Can you work these out from the model? Positions are in its coordinate system, mm. Face numbers are marked on the shaded views. A direction names the side the tool comes from. Round coordinates to 2 decimals unless told otherwise and drop trailing zeros. Write each loop counter-clockwise with the first axis right and the second up, starting at its lowest first coordinate (ties: lowest second). Pieces come first, ordered by that corner, then holes. Notation, with made-up numbers: M 32.5,66 L 80.5,66 A32 cw 80.5,104 Z; hole C 4,42 d10. An arc over 180 degrees is marked long. Answer in a Markdown table with one row per item. Add a question column.
(1) If I drill on probe 1 along Y at (x, z) = (0, 0.25); probe 2 along Y at (x, z) = (0, 0.1); probe 3 along Z at (x, y) = (-1.25, -5), over which ranges is the centre line in solid material (lowest first)?
(2) I'm going to push flat-ended pins straight in: pin 1 (3.5 mm diameter, centred on x = 0, y = -2.8, fed in from +Z); pin 2 (0.6 mm diameter, centred on x = 1, z = 1, fed in from -Y); pin 3 (1 mm diameter, centred on y = -2.5, z = 1.5, fed in from -X). Where does each tip first touch, or does it pass through?
(3) Suppose I cut it at B-B, the plane z = 0.15. Write out the boundary of the cut face in (x, y) (3 decimals), then the cut area to 3 significant figures.
(4) For the marked faces 5 and 6, which set-ups out of +Z, -Z, +X, -X, +Y, -Y let a thin tool reach every point of the face, with its end or its side?
(5) Suppose I cut it at D-D, the plane z = 0.8. Write out the boundary of the cut face in (x, y) (3 decimals).
(6) Suppose I cut it at A-A, the plane y = -2.8. Write out the boundary of the cut face in (x, z) (3 decimals).
(7) Suppose I cut it at C-C, the plane x = 0. Write out the boundary of the cut face in (y, z).
(8) If we mould it in two halves opening along Y, with no side actions, what happens to the marked faces 1, 2, 3 and 4? For each: released by +Y, released by -Y, zero draft, split by the parting line, or undercut.
from build123d import *

# Parameters (mm, degrees)
F1_DEPTH = 3.175
F2_R     = 0.8
F4_D     = 3.2


with BuildPart() as f1:
    # F0 (on Right) → F1 (new body, symmetric)
    with BuildSketch(Plane.YZ):
        with BuildLine():
            Line((-5.4, 0), (0, 0))
            Line((0, 0), (0, 0.4))
            Line((0, 0.4), (-5.4, 0.4))
            ThreePointArc((-5.4, 0.4), (-5.541421, 0.458579), (-5.6, 0.6))
            Line((-5.6, 0.6), (-5.6, 1.4))
            ThreePointArc((-5.6, 1.4), (-6.063558, 2.243937), (-7.02446, 2.305447))
            Line((-7.02446, 2.305447), (-11.089105, 0.4))
            Line((-11.089105, 0.4), (-12.33, 0.4))
            Line((-12.33, 0.4), (-12.33, 0))
            Line((-12.33, 0), (-11, 0))
            Line((-11, 0), (-6.854676, 1.943268))
            ThreePointArc((-6.854676, 1.943268), (-6.278135, 1.906362), (-6, 1.4))
            Line((-6, 1.4), (-6, 0.6))
            ThreePointArc((-6, 0.6), (-5.824264, 0.175736), (-5.4, 0))
        make_face()
    extrude(amount=F1_DEPTH, both=True)

    # F2
    f2_edges = [f1.edges().sort_by_distance(p)[0] for p in [
        (3.175, -12.33, 0.2),
        (-3.175, -12.33, 0.2),
        (3.175, 0, 0.2),
        (-3.175, 0, 0.2),
    ]]
    fillet(f2_edges, radius=F2_R)

    # F4 (through all)
    with Locations(Plane.XY.offset(0.4)):
        with Locations((0, -2.8)):
            Hole(F4_D / 2)


solid = f1.part
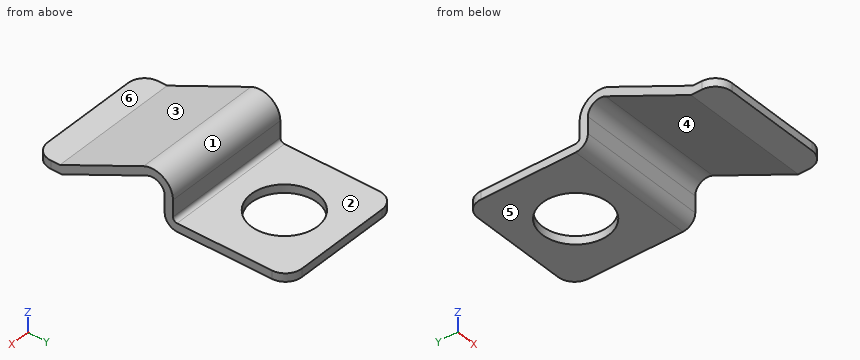
Calculated:
| question | item | result |
|---|---|---|
| 1 | probe 1 | -12.33 to -10.47, -5.89 to -4.4, -1.2 to 0 |
| 1 | probe 2 | -12.33 to -10.79, -5.73 to -4.4, -1.2 to 0 |
| 1 | probe 3 | 0 to 0.4 |
| 2 | pin 1 | z = 0.4 |
| 2 | pin 2 | y = -10.45 |
| 2 | pin 3 | through |
| 3 | outline | M -3.175,-11.53 A0.8 ccw -2.375,-12.33 L 2.375,-12.33 A0.8 ccw 3.175,-11.53 L 3.175,-10.68 L -3.175,-10.68 Z; M -3.175,-5.797 L 3.175,-5.797 L 3.175,-0.8 A0.8 ccw 2.375,0 L -2.375,0 A0.8 ccw -3.175,-0.8 Z; hole C 0,-2.8 d3.2 |
| 3 | area | 38.7 mm² |
| 4 | face 5 | -Z, +X, -X, +Y, -Y |
| 4 | face 6 | +Z, +X, -X, -Y |
| 5 | outline | M -3.175,-10.236 L 3.175,-10.236 L 3.175,-9.293 L -3.175,-9.293 Z; M -3.175,-6 L 3.175,-6 L 3.175,-5.6 L -3.175,-5.6 Z |
| 6 | outline | M -3.175,0 L -1.6,0 L -1.6,0.4 L -3.175,0.4 Z; M 1.6,0 L 3.175,0 L 3.175,0.4 L 1.6,0.4 Z |
| 7 | outline | M -12.33,0 L -11,0 L -6.85,1.94 A0.6 cw -6,1.4 L -6,0.6 A0.6 ccw -5.4,0 L -4.4,0 L -4.4,0.4 L -5.4,0.4 A0.2 cw -5.6,0.6 L -5.6,1.4 A1 ccw -7.02,2.31 L -11.09,0.4 L -12.33,0.4 Z; M -1.2,0 L 0,0 L 0,0.4 L -1.2,0.4 Z |
| 8 | face 1 | split by the parting line |
| 8 | face 2 | zero draft |
| 8 | face 3 | released by -Y |
| 8 | face 4 | undercut |
